Autodesk Inventor part; units mm, degrees
ref_plane "YZ Plane" through (0, 0, 0) normal (1, 0, 0) x (0, 1, 0)
ref_plane "XZ Plane" through (0, 0, 0) normal (0, 1, 0) x (-1, 0, 0)
ref_plane "XY Plane" through (0, 0, 0) normal (0, 0, 1) x (1, 0, 0)
sketch "Sketch1" plane through (0, 0, 0) normal (0, 0, 1) x (1, 0, 0)
  circle A0 centre (0, 0) radius 14.2875
  dimension "d0" = 28.575
extrude "Extrusion1" add sketch "Sketch1" along normal blind 1.5875
sketch "Sketch2" plane through (0, 0, 1.5875) normal (0, 0, 1) x (1, 0, 0)
  point P0 (0, 0)
  point P1 (0, 9.017)
  point P2 (9.017, 0)
  point P3 (0, -9.017)
  point P4 (-9.017, 0)
  dimension "d3" = 9.017
  dimension "d4" = 9.017
  dimension "d5" = 9.017
  dimension "d6" = 9.017
hole "Hole1" at (0, 9.017, 1.5875) at (9.017, 0, 1.5875) at (0, -9.017, 1.5875) at (-9.017, 0, 1.5875) direction (0, 0, -1) diameter 4.4958 depth 12.2936 tip angle 118
sketch "Sketch3" plane through (0, 0, 1.5875) normal (0, 0, 1) x (1, 0, 0)
  circle A0 centre (0, 0) radius 2.54
  dimension "d14" = 5.08
extrude "Extrusion2" cut sketch "Sketch3" against normal blind 1.5875
chamfer "Chamfer1" distance 1.5875 angle 45 1 edges at (-2.54, 0, 1.5875)
properties part number "piercable_septum_clamp"
Here's how the part is built. I have some questions about the finished solid (model axes, mm). Round coordinates to 2 decimals unless told otherwise and drop trailing zeros. Order: outer loops, then holes, each group sorted by start corner. A loop starts at its lowest first (then second) coordinate and runs counter-clockwise, first axis right, second up. Notation, with made-up numbers: M 13.25,86 L 62.25,86 A13 ccw 62.25,104 Z; hole C 42,27.25 d6. An arc over 180 degrees is marked long. Answer in a Markdown table with one row per item.
Item 1: Imagine slicing it at D-D, the plane y = 9.5. Write out the boundary of the cut face in (x, z).
A:
| item | result |
|---|---|
| outline | M -10.67,0 L -2.2,0 L -2.2,1.59 L -10.67,1.59 Z; M 2.2,0 L 10.67,0 L 10.67,1.59 L 2.2,1.59 Z |
Item 2: Thinking about a two-plate mould opening in X: for faces 1 (the face through (11.01, -1.04, 0.78)), 2 (the face through (0, -3, 0)), 3 (the face through (-14.274, -0.628, 0.783)), which applies, +X half, -X half, draft (parallel to the pull), parting line (faces both ways), or undercut?
A:
| item | result |
|---|---|
| face 1 | undercut |
| face 2 | draft |
| face 3 | parting line |
Item 3: Imagine slicing it at C-C, the plane z = 0.95. Write out the boundary of the cut face in (x, y) (1 decimal), and give its area (3 significant figures).
A:
| item | result |
|---|---|
| outline | C 0,0 d28.6; hole C -9,0 d4.5; hole C 0,0 d7; hole C 0,-9 d4.5; hole C 0,9 d4.5; hole C 9,0 d4.5 |
| area | 540 mm2 |
Item 4: If I drill on L1, parallel to Y at x = 1.75, z = 1.35; L2, parallel to Y at x = 0.25, z = 1.1; L3, parallel to Y at x = -9, z = 1.55, over which ranges is the centre line in solid material (lowest first)? Write a range as from..to.
A:
| item | result |
|---|---|
| L1 | y = -14.18..-10.43, -7.61..-3.47, 3.47..7.61, 10.43..14.18 |
| L2 | y = -14.29..-11.25, -6.78..-3.63, 3.63..6.78, 11.25..14.29 |
| L3 | y = -11.1..-2.25, 2.25..11.1 |
Item 5: Imagine slicing it at A-A, the plane x = 0. State how many separate pieces and enclosed holes the cut face has, and give its area (3 significant figures).
A:
| item | result |
|---|---|
| separate pieces | 4 |
| enclosed holes | 0 |
| area | 20.5 mm2 |
